Verification items for this drawing (mm, ordinates from the low corner). A direction names the side the tool comes from. Coordinates: 2 decimals unless noted, no trailing zeros. Loops run counter-clockwise (first coordinate to the right, second up) from the corner with the lowest first, then second, coordinate; pieces in that order, holes last. Notation, with made-up numbers: (-31.5, 10) -> (-25.5, 10) arc R9 cw to (-25.5, 26) -> close; hole circle Ø4 at (31.25, 42.25). An arc over 180 degrees is marked (long way). Write item = value, one per line.
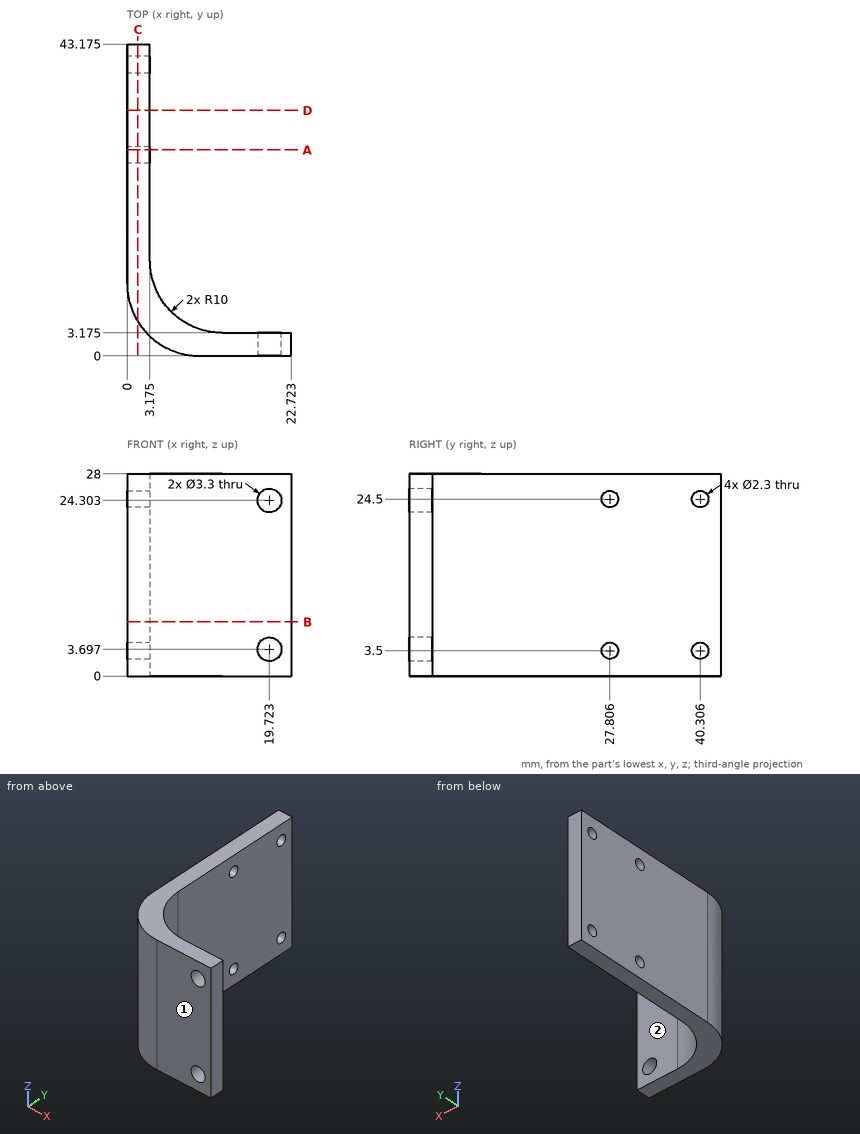
1) Material ranges on line 1 (Y direction, x = 1.6, z = 24.5) (1 decimal); line 2 (Y direction, x = 1.4, z = 3.5) (1 decimal); line 3 (X direction, y = 15, z = 8.75) (1 decimal), recorded low to high.
Ans:
line_1 = 4.6 to 26.7, 29 to 39.2, 41.5 to 43.2
line_2 = 4.9 to 26.7, 29 to 39.2, 41.5 to 43.2
line_3 = 0 to 3.2
2) Depth check by flat-ended pin: pin 1 Ø8 at (x, y) = (7.5, 29) entering from +Z; pin 2 Ø1 at (x, z) = (4.5, 8.5) entering from +Y; pin 3 Ø10.5 at (x, z) = (18.5, 7.5) entering from +Y (3 decimals); pin 4 Ø5 at (x, z) = (6, 13) entering from -Y. Enter the tip coordinate at first touch or a pass-through.
Ans:
pin_1 = through
pin_2 = 9.2
pin_3 = 3.175
pin_4 = 0.11
3) Sectioned sample at A-A, the plane y = 28.5. Record the cut outline in (x, z) (1 decimal).
Ans:
outline = (0, 0) -> (3.2, 0) -> (3.2, 2.6) -> (0, 2.6) -> close; (0, 4.4) -> (3.2, 4.4) -> (3.2, 23.6) -> (0, 23.6) -> close; (0, 25.4) -> (3.2, 25.4) -> (3.2, 28) -> (0, 28) -> close
4) Sectioned sample at B-B, the plane z = 7.5. Record the cut outline in (x, y) (1 decimal), plus the area to 3 significant figures.
Ans:
outline = (0, 10) arc R10 ccw to (10, 0) -> (22.7, 0) -> (22.7, 3.2) -> (13.2, 3.2) arc R10 cw to (3.2, 13.2) -> (3.2, 43.2) -> (0, 43.2) -> close
area = 199 mm2
5) Tool access check on the marked faces 1 and 2. Record the directions out of +Z, -Z, +X, -X, +Y, -Y that give a thin tool (end or side, any length) a straight path to the whole face; none if there is none.
Ans:
face_1 = +Z, -Z, +X, -X, -Y
face_2 = +Z, -Z, +X, +Y
6) Sectioned sample at C-C, the plane x = 1.5. Count the separate pieces of the cut face and the enclosed holes in it, plus the area to 3 significant figures.
Ans:
separate_pieces = 1
enclosed_holes = 4
area = 1,060 mm2
7) Sectioned sample at D-D, the plane y = 34. Record the cut outline in (x, z) (1 decimal), plus the area to 3 significant figures.
Ans:
outline = (0, 0) -> (3.2, 0) -> (3.2, 28) -> (0, 28) -> close
area = 88.9 mm2
